Source: CAD feature listing. Evaluate the final solid. Frame: model axes, mm. Face numbers are marked on the shaded views. Give positions to 0.01 mm unless a question says otherwise; leave off trailing zeros. Loops run counter-clockwise (first coordinate to the right, second up) from the corner with the lowest first, then second, coordinate; pieces in that order, holes last. Notation, with made-up numbers: (56.25, 60) - (81.25, 60) arc R35 cw to (81.25, 95) - close; hole circle Ø6 at (57, -0.75). An arc over 180 degrees is marked (long way). Write each question's results on one line, items separated by ' | '. Start each with the question number.
(1) Material intervals for line 1 along Y through (x, z) = (-52.5, -2.5) (3 decimals); line 2 along Y through (x, z) = (-53, -4.25) (3 decimals); line 3 along X through (y, z) = (-83, -3.25), sorted ascending. Write a range as [from, to].
(2) Cut plane A-A on y = -92.71. Return the cut outline in (x, z), then the cut area to 3 significant figures.
(3) Pull-direction query (Y, two-part tool) for the marked faces 1, 2 and 3; classes: pulls with the +Y half, pulls with the -Y half, needs draft (parallel to the pull), parting line crosses it, or undercut.
(4) Cut plane B-B on z = -2.5. Return the cut outline in (x, y) (3 decimals).
(5) Cut plane C-C on x = -43. Give the number of separate pieces and of enclosed holes in the cut face, then the cut area to 3 significant figures.
from build123d import *

# Parameters (mm, degrees)
F0_W     = 38.1
F0_H     = 101.6
F1_DEPTH = 6.35
F2_D     = 22
F3_D     = 4.3053


with BuildPart() as f1:
    # F0 (on Top) → F1 (new body)
    with BuildSketch(Plane.XY):
        with Locations((-51.9482906996, -46.355)):
            Rectangle(F0_W, F0_H)
    extrude(amount=-F1_DEPTH)

    # F2 (through all)
    with Locations(Plane.XY):
        with Locations((-51.9482906996, -10.033), (-51.9482906996, -82.677)):
            Hole(F2_D / 2)

    # F3 (through all)
    with Locations(Plane.XY):
        with Locations((-39.2482906996, 0), (-39.2482906996, -92.71)):
            Hole(F3_D / 2)


solid = f1.part
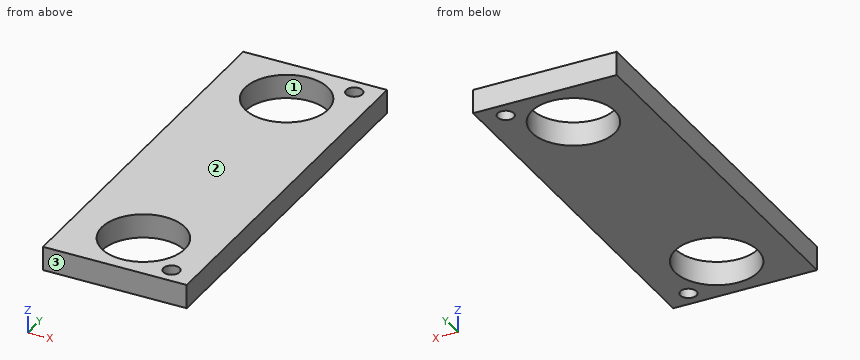
Ans:
1) line 1: [-97.155, -93.663], [-71.691, -21.019], [0.953, 4.445] | line 2: [-97.155, -93.627], [-71.727, -20.983], [0.917, 4.445] | line 3: [-71, -62.94], [-40.95, -32.9]
2) outline: (-71, -6.35) - (-56.46, -6.35) - (-56.46, 0) - (-71, 0) - close; (-47.44, -6.35) - (-41.4, -6.35) - (-41.4, 0) - (-47.44, 0) - close; (-37.1, -6.35) - (-32.9, -6.35) - (-32.9, 0) - (-37.1, 0) - close | area: 157 mm^2
3) face 1: undercut | face 2: needs draft | face 3: pulls with the -Y half
4) outline: (-70.998, -97.155) - (-32.898, -97.155) - (-32.898, 4.445) - (-70.998, 4.445) - close; hole circle Ø22 at (-51.948, -82.677); hole circle Ø22 at (-51.948, -10.033); hole circle Ø4.305 at (-39.248, -92.71); hole circle Ø4.305 at (-39.248, 0)
5) separate pieces: 3 | enclosed holes: 0 | area: 483 mm^2
